The model under review builds one solid part; all positions refer to its coordinate system, in mm. Face numbers are marked on the shaded views. A direction names the side the tool comes from. Give positions to 0.01 mm unless a question says otherwise; leave off trailing zeros. Order: outer loops, then holes, each group sorted by start corner. A loop starts at its lowest first (then second) coordinate and runs counter-clockwise, first axis right, second up.
```python
from build123d import *

# Parameters (mm, degrees)
BLANKSKE_W          = 12
BLANKSKE_H          = 4.7
BLANK_DEPTH         = 8
TOOTHCUTSIM_DEPTH   = 16.16871781
TEETHCUTS_COUNT     = 6
TEETHCUTS_PITCH     = 2.199114855
SKETCH1_W           = 12
SKETCH1_H           = 2
BOSS_EXTRUDE1_DEPTH = 5
SKETCH2_W           = 0.75
SKETCH2_H           = 8
CUT_EXTRUDE1_DEPTH  = 5
SKETCH3_W           = 3.8
SKETCH3_H           = 2.8
BOSS_EXTRUDE2_DEPTH = 23
SKETCH4_W           = 3.8
SKETCH4_H           = 1.4
CUT_EXTRUDE2_DEPTH  = 3


with BuildPart() as part:
    # BlankSke → Blank (new body)
    with BuildSketch(Plane.XY):
        with Locations((6, 2.35)):
            Rectangle(BLANKSKE_W, BLANKSKE_H)
    extrude(amount=-BLANK_DEPTH)

    # TooCutSkeSim → ToothCutSim (cut, through all)
    with BuildSketch(Plane.XY):
        Polygon((0.312304759, 3.125), (-0.312304759, 3.125), (-0.894802722, 4.7254), (0.894802722, 4.7254), align=None)
    toothcutsim = extrude(amount=-TOOTHCUTSIM_DEPTH, mode=Mode.SUBTRACT)

    # TeethCuts: ToothCutSim ×6
    with Locations(*[(i * TEETHCUTS_PITCH, 0, 0) for i in range(1, TEETHCUTS_COUNT)]):
        add(toothcutsim, mode=Mode.SUBTRACT)

    # Sketch1 → Boss-Extrude1 (add)
    with BuildSketch(Plane.XZ):
        with Locations((6, -1)):
            Rectangle(SKETCH1_W, SKETCH1_H)
        with Locations((6, -7)):
            Rectangle(SKETCH1_W, SKETCH1_H)
    extrude(amount=-BOSS_EXTRUDE1_DEPTH)

    # Sketch2 → Cut-Extrude1 (cut)
    with BuildSketch(Plane(origin=(0, 0, 0), x_dir=(1, 0, 0), z_dir=(0, 1, 0))):
        with Locations((11.625, 4)):
            Rectangle(SKETCH2_W, SKETCH2_H)
    extrude(amount=CUT_EXTRUDE1_DEPTH, mode=Mode.SUBTRACT)

    # Sketch3 → Boss-Extrude2 (add)
    with BuildSketch(Plane(origin=(0, 0, 0), x_dir=(0, 0, -1), z_dir=(1, 0, 0))):
        with Locations((4, 1.5)):
            Rectangle(SKETCH3_W, SKETCH3_H)
    extrude(amount=-BOSS_EXTRUDE2_DEPTH)

    # Sketch4 → Cut-Extrude2 (cut)
    with BuildSketch(Plane.ZY.offset(23)):
        with Locations((-4, 0.8)):
            Rectangle(SKETCH4_W, SKETCH4_H)
    extrude(amount=-CUT_EXTRUDE2_DEPTH, mode=Mode.SUBTRACT)


solid = part.part
```
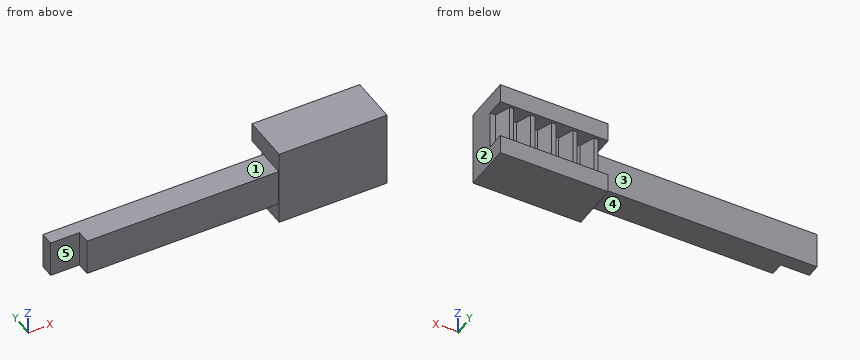
1. Take a section at C-C (x = -4.5). Write out the cut boundary in (y, z), and give its area (3 significant figures).
2. Take a section at A-A (y = 1.85). Write out the cut boundary in (x, z), and give its area (3 significant figures).
3. Draft analysis for pull direction X (two halves, no side actions). For the marked faces 1 and 2, state which applies: pulls with the +X half, pulls with the -X half, needs draft (parallel to the pull), parting line crosses it, or undercut.
4. For the marked faces 3, 4 and 5, list the 3-axis set-ups (+Z, -Z, +X, -X, +Y, -Y) from which the entire face can be reached by the end or side of a thin tool; tool diameter is ignored.
5. To check wall thickness, follow line 1 (Z direction, x = 0.5, y = 4.25); line 2 (X direction, y = 3.3, z = -4.75); line 3 (X direction, y = 1.8, z = -6.5). State the ranges of each line that lie inside material, in increasing order.
6. Insertion check: pin 1 (0.5 mm diameter, centred on x = 10, z = -4, fed in from +Y); pin 2 (3 mm diameter, centred on y = 4, z = -7, fed in from -X); pin 3 (0.5 mm diameter, centred on x = 11, z = -4.5, fed in from +Y) (3 decimals). Each pin has a flat end and moves straight along its axis. Give the tip position at first contact, or say it passes through.
7. Take a section at D-D (y = 3.7). Write out the cut boundary in (x, z).
Answer:
1. outline: (0.1, -5.9) - (2.9, -5.9) - (2.9, -2.1) - (0.1, -2.1) - close
1. area: 10.6 mm2
2. outline: (-23, -5.9) - (0, -5.9) - (0, -8) - (11.25, -8) - (11.25, 0) - (0, 0) - (0, -2.1) - (-23, -2.1) - close
2. area: 177 mm2
3. face 1: needs draft
3. face 2: pulls with the +X half
4. face 3: +Z, -Z, -X, +Y
4. face 4: -Z, -X, +Y, -Y
4. face 5: +Z, -Z, -X, -Y
5. line 1: z = -8 to -6, -2 to 0
5. line 2: x = 0.38 to 1.82, 2.58 to 4.02, 4.77 to 6.22, 6.97 to 8.42, 9.17 to 10.62
5. line 3: x = 0 to 11.25
6. pin 1: stops at y = 4.7
6. pin 2: stops at x = 0
6. pin 3: stops at y = 3.125
7. outline: (0, -8) - (11.25, -8) - (11.25, -6) - (10.47, -6) - (10.47, -2) - (11.25, -2) - (11.25, 0) - (0, 0) - (0, -2) - (0.52, -2) - (0.52, -6) - (0, -6) - close; hole (1.68, -6) - (2.72, -6) - (2.72, -2) - (1.68, -2) - close; hole (3.88, -6) - (4.92, -6) - (4.92, -2) - (3.88, -2) - close; hole (6.08, -6) - (7.12, -6) - (7.12, -2) - (6.08, -2) - close; hole (8.27, -6) - (9.32, -6) - (9.32, -2) - (8.27, -2) - close
